```python
from build123d import *

# Parameters (mm, degrees)
F0_W     = 1828.8
F0_H     = 1828.8
F1_DEPTH = 152.4
F3_DEPTH = 1828.801
F4_DEPTH = 1828.8


with BuildPart() as f1:
    # F0 (on Top) → F1 (new body)
    with BuildSketch(Plane.XY):
        Rectangle(F0_W, F0_H)
    extrude(amount=F1_DEPTH)

    # F2 (on face) → F3 (cut, through all)
    with BuildSketch(Plane.XZ.offset(914.4)):
        Polygon((914.4, 152.4), (-914.4, 152.4), (914.4, 0), align=None)
    extrude(amount=-F3_DEPTH, mode=Mode.SUBTRACT)

    # F2 (on face) → F4 (join, through all)
    with BuildSketch(Plane.XZ.offset(914.4)):
        Polygon((914.4, 0), (-914.4, 152.4), (-928.276584, -14.119007), (900.523416, -166.519007), align=None)
    extrude(amount=-F4_DEPTH)


solid = f1.part
```
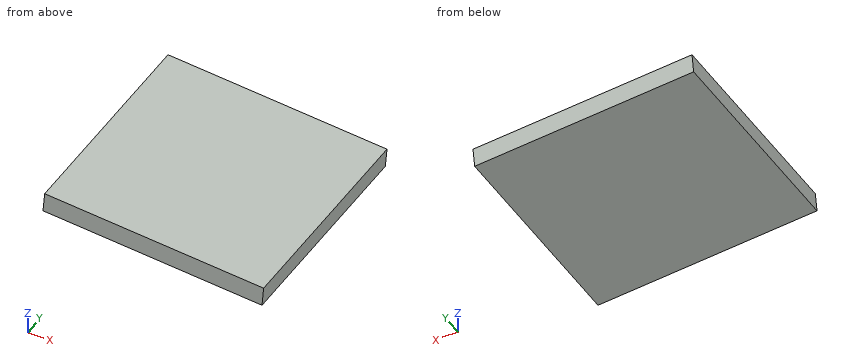
Input: part model. Units: mm. Frame: model coordinates. Round coordinates to 2 decimals unless told otherwise and drop trailing zeros. Order: outer loops, then holes, each group sorted by start corner. A loop starts at its lowest first (then second) coordinate and runs counter-clockwise, first axis right, second up. Notation, with made-up numbers: (18.25, 51) - (62.25, 51) arc R26 ccw to (62.25, 81) - close; hole circle Ø7 at (35, 15). An arc over 180 degrees is marked (long way). Answer in a Markdown table with one row per item.
Item 1: Section query A-A (y = -499). Return the cut outline in (x, z).
Model answer:
| item | result |
|---|---|
| outline | (-928.28, -14.12) - (900.52, -166.52) - (914.4, 0) - (-914.4, 152.4) - close |
Item 2: Line query: line 1 (Z direction, x = 814.5, y = -529.5) (3 decimals); line 2 (Z direction, x = -848, y = -621). Output: solid intervals per line, ascending.
Model answer:
| item | result |
|---|---|
| line 1 | z = -159.35 to 8.325 |
| line 2 | z = -20.81 to 146.87 |
Item 3: Pin query (flat end, axial travel): pin 1 (8 mm diameter, centred on y = 118, z = 27.5, fed in from -X); pin 2 (12 mm diameter, centred on x = 621.5, y = 311.5, fed in from +Z); pin 3 (2 mm diameter, centred on x = -364.5, y = 587, fed in from -Z). Return the tip coordinate at first contact, or that it passes through.
Model answer:
| item | result |
|---|---|
| pin 1 | stops at x = -925.14 |
| pin 2 | stops at z = 24.91 |
| pin 3 | stops at z = -61.18 |
Item 4: Section query B-B (z = 78). Return the cut outline in (x, y).
Model answer:
| item | result |
|---|---|
| outline | (-920.6, -914.4) - (-21.6, -914.4) - (-21.6, 914.4) - (-920.6, 914.4) - close |
